```python
from build123d import *

# Parameters (mm, degrees)
SKETCH1_W                  = 17
SKETCH1_H                  = 22
BOSS_EXTRUDE1_DEPTH        = 29.2
SKETCH3_R                  = 4
BOSS_EXTRUDE2_DEPTH        = 2.94
BOSS_EXTRUDE2_TAPER        = 10
SKETCH4_R                  = 4.5
BOSS_EXTRUDE3_DEPTH        = 8.6
CHAMFER1_SIZE              = 0.5
SKETCH13_R                 = 3.25
CUT_EXTRUDE1_DEPTH         = 29
SKETCH14_W                 = 0.4
SKETCH14_H                 = 1.2
BOSS_EXTRUDE4_DEPTH        = 3.25
LPATTERN1_COUNT            = 2
LPATTERN1_PITCH            = 16.5
CHAMFER1_OF_LPATTERN1_SIZE = 0.5
LPATTERN2_COUNT            = 2
LPATTERN2_PITCH            = 3.17
LPATTERN2_COUNT_DIR2       = 2
LPATTERN2_PITCH_DIR2       = 1.27
SKETCH15_R                 = 2
CUT_EXTRUDE2_DEPTH         = 2


with BuildPart() as part:
    # Sketch1 → Boss-Extrude1 (new body)
    with BuildSketch(Plane(origin=(0, 0, 0), x_dir=(1, 0, 0), z_dir=(0, 1, 0))):
        with Locations((-7.350772662, 1.631732914)):
            Rectangle(SKETCH1_W, SKETCH1_H)
    extrude(amount=BOSS_EXTRUDE1_DEPTH)

    # Sketch3 → Boss-Extrude2 (add)
    with BuildSketch(Plane(origin=(0, 0, -12.631732914), x_dir=(-1, 0, 0), z_dir=(0, 0, -1))):
        with Locations((8.650772662, 6.5)):
            Circle(SKETCH3_R)
    boss_extrude2 = extrude(amount=BOSS_EXTRUDE2_DEPTH, taper=BOSS_EXTRUDE2_TAPER)

    # Sketch4 → Boss-Extrude3 (add)
    with BuildSketch(Plane.XY.offset(9.368267086)):
        with Locations(Location((-8.650772662, 6.5, 0), (0, 0, 180))):
            Circle(SKETCH4_R)
    boss_extrude3 = extrude(amount=BOSS_EXTRUDE3_DEPTH)

    # Chamfer1
    chamfer1_edges = [part.edges().sort_by_distance(p)[0] for p in [
        (-4.150772662, 6.5, 17.968267086),
    ]]
    chamfer(chamfer1_edges, length=CHAMFER1_SIZE)

    # Sketch13 → Cut-Extrude1 (cut)
    with BuildSketch(Plane.XY.offset(17.968267086)):
        with Locations((-8.650772662, 6.5)):
            Circle(SKETCH13_R)
    cut_extrude1 = extrude(amount=-CUT_EXTRUDE1_DEPTH, mode=Mode.SUBTRACT)

    # Sketch14 → Boss-Extrude4 (add)
    with BuildSketch(Plane.XZ):
        with Locations((-13.900772662, 4.758267086)):
            Rectangle(SKETCH14_W, SKETCH14_H)
        with Locations((-2.470772662, 4.758267086)):
            Rectangle(SKETCH14_W, SKETCH14_H)
        with Locations((-2.470772662, -7.931732914)):
            Rectangle(SKETCH14_W, SKETCH14_H)
        with Locations((-13.900772662, -7.931732914)):
            Rectangle(SKETCH14_W, SKETCH14_H)
    boss_extrude4 = extrude(amount=BOSS_EXTRUDE4_DEPTH)

    # LPattern1: Boss-Extrude2, Boss-Extrude3, Cut-Extrude1 ×2
    with Locations(*[(0, i * LPATTERN1_PITCH, 0) for i in range(1, LPATTERN1_COUNT)]):
        add(boss_extrude2)
        add(boss_extrude3)
        add(cut_extrude1, mode=Mode.SUBTRACT)

    # Chamfer1 of LPattern1
    chamfer1_of_lpattern1_edges = [part.edges().sort_by_distance(p)[0] for p in [
        (-4.150772662, 23, 17.968267086),
    ]]
    chamfer(chamfer1_of_lpattern1_edges, length=CHAMFER1_OF_LPATTERN1_SIZE)

    # LPattern2: Boss-Extrude4 2 × 2, 2 skipped
    with Locations(*[(j * LPATTERN2_PITCH_DIR2, 0, -i * LPATTERN2_PITCH) for i in range(LPATTERN2_COUNT) for j in range(LPATTERN2_COUNT_DIR2) if (i, j) not in ((0, 0), (0, 1), (1, 0))]):
        add(boss_extrude4)

    # Sketch15 → Cut-Extrude2 (cut)
    with BuildSketch(Plane.XY.offset(9.368267086)):
        with Locations((-8.650772662, 14.75)):
            Circle(SKETCH15_R)
    extrude(amount=-CUT_EXTRUDE2_DEPTH, mode=Mode.SUBTRACT)


solid = part.part
```
For this review, take the finished solid that the model builds, in its own axes (mm). A direction names the side the tool comes from. Coordinates: 2 decimals unless noted, no trailing zeros. Loops run counter-clockwise (first coordinate to the right, second up) from the corner with the lowest first, then second, coordinate; pieces in that order, holes last. Notation, with made-up numbers: (32, -19.5) -> (53, -19.5) arc R16 ccw to (53, -3.5) -> close; hole circle Ø7 at (45.5, 36). An arc over 180 degrees is marked (long way). Return JSON: item names as keys, results as strings. Group by question number.
(1) For pin 1 Ø1.3 at (y, z) = (-1, 1.5) entering from -X; pin 2 Ø10 at (x, z) = (-2, 8.5) entering from -Y; pin 3 Ø1.3 at (y, z) = (-2, 2) entering from +X; pin 4 Ø5 at (x, z) = (-13, 13) entering from -Y, all flat-tipped, find the tip position at first contact; note any pin that passes through.
(2) Consider section B-B, the plane z = 15.5. Give the boundary of the cut face in (x, y), plus the area to 3 significant figures.
(3) Tool access review of faces 4 (the flat face through (-12.831, -2, 2)), 5 (the flat face through (-7, 14, -12.632)), 6 (the flat face through (-12.431, -2, -11)), 7 (the flat face through (-6, 14, 9.368)): name each direction out of +Z, -Z, +X, -X, +Y, -Y from which nothing blocks a thin tool from reaching the whole face with its end or side.
(4) Consider section A-A, the plane y = 14.75. Give the boundary of the cut face in (x, z).
(5) Mouldability with a two-part tool opening along X and no side actions: class faces 1 (the conical face through (-5.777, 4.296, -14.776)), 2 (the flat face through (-2.671, -2, -8)), 3 (the flat face through (-14.101, -2, 5)) as pulls with the +X half, pulls with the -X half, needs draft (parallel to the pull), parting line crosses it, or undercut.
(6) To check wall thickness, follow L1, parallel to Y at x = -8.75, z = -8; L2, parallel to Y at x = -11.5, z = 3; L3, parallel to Y at x = -10, z = 16. State the ranges of each line that lie inside material, in increasing order.
(7) Consider section C-C, the plane z = 0.5. Give the boundary of the cut face in (x, y), plus the area to 3 significant figures.
(8) Consider section D-D, the plane x = -3.5. Give the boundary of the cut face in (y, z).
Results below:
{
 "1": {"pin 1": "stops at x = -12.83", "pin 2": "stops at y = -3.25", "pin 3": "stops at x = -1", "pin 4": "stops at y = 2.4"},
 "2": {"outline": "circle Ø9 at (-8.65, 6.5); circle Ø9 at (-8.65, 23); hole circle Ø6.5 at (-8.65, 6.5); hole circle Ø6.5 at (-8.65, 23)", "area": "60.9 mm2"},
 "3": {"face 4": "+Z, -Z, -X, -Y", "face 5": "-Z", "face 6": "+Z, -Z, -Y", "face 7": "+Z"},
 "4": {"outline": "(-15.85, -12.63) -> (1.15, -12.63) -> (1.15, 9.37) -> (-6.65, 9.37) -> (-6.65, 7.37) -> (-10.65, 7.37) -> (-10.65, 9.37) -> (-15.85, 9.37) -> close"},
 "5": {"face 1": "parting line crosses it", "face 2": "undercut", "face 3": "pulls with the -X half"},
 "6": {"L1": "y = 0 to 3.25, 9.75 to 19.75, 26.25 to 29.2", "L2": "y = 0 to 4.94, 8.06 to 21.44, 24.56 to 29.2", "L3": "y = 2.21 to 3.54, 9.46 to 10.79, 18.71 to 20.04, 25.96 to 27.29"},
 "7": {"outline": "(-15.85, 0) -> (1.15, 0) -> (1.15, 29.2) -> (-15.85, 29.2) -> close; hole circle Ø6.5 at (-8.65, 6.5); hole circle Ø6.5 at (-8.65, 23)", "area": "430 mm2"},
 "8": {"outline": "(0, -12.63) -> (29.2, -12.63) -> (29.2, 9.37) -> (0, 9.37) -> close"}
}
